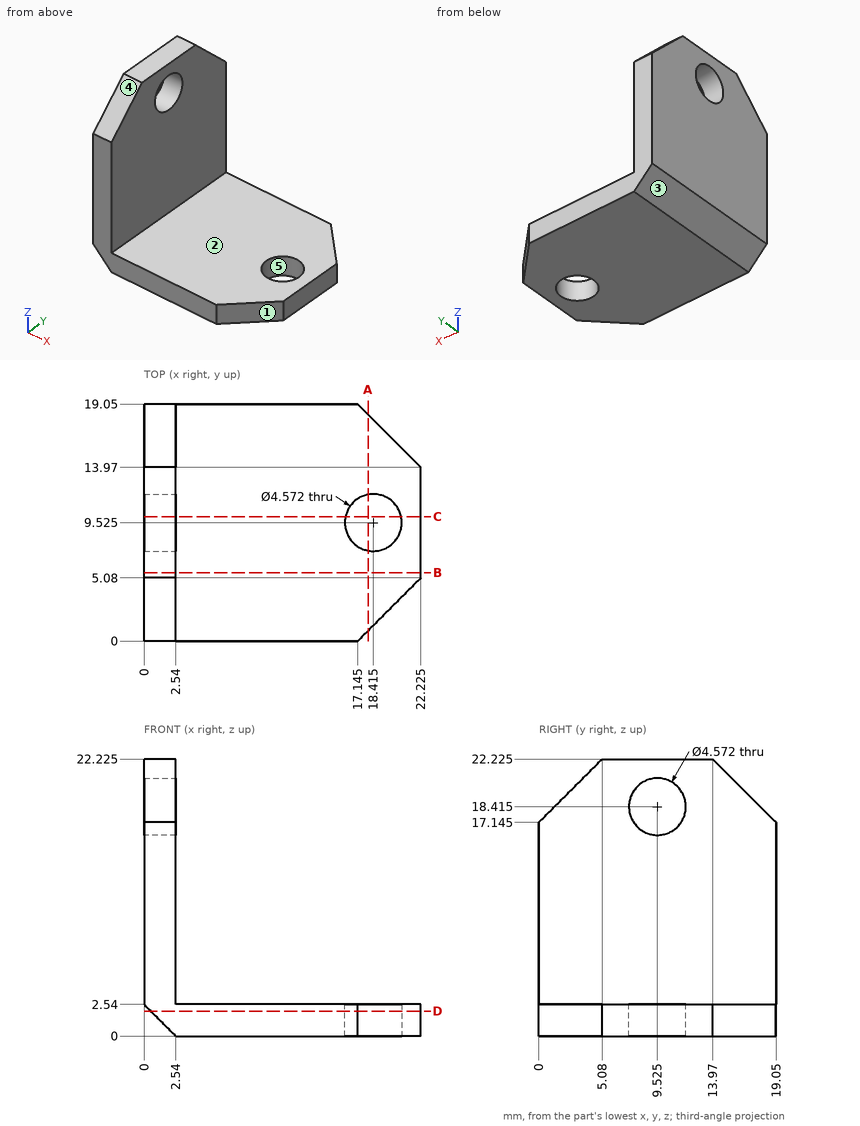
For this review, use the dimensioned drawing (mm, ordinates from the lowest corner) and the shaded views. A direction names the side the tool comes from. Give positions to 0.01 mm unless a question says otherwise; leave off trailing zeros. Order: outer loops, then holes, each group sorted by start corner. A loop starts at its lowest first (then second) coordinate and runs counter-clockwise, first axis right, second up. Notation, with made-up numbers: M -4,53 L 24,53 A21 ccw 24,77 Z; hole C -6,82 d11. An arc over 180 degrees is marked long. One line per question, with ' | ' between items. Start each with the question number.
1) Wall thickness on L1, parallel to Z at x = 8.75, y = 6; L2, parallel to X at y = 9.25, z = 1.5 (3 decimals): over which ranges is each line inside the solid? List them lowest first. Write a range as from..to.
2) Consider section C-C, the plane y = 10. Give the boundary of the cut face in (x, z) (3 decimals), then the cut area to 3 significant figures.
3) Clearance check with flat-ended pins moving along their axes: P1, Ø10, axis at x = 18.5, y = 15, coming from the +Z side; P2, Ø5.5, axis at y = 11.5, z = 8.5, coming from the +X side. State where each tip first meets the part, or that it passes through.
4) Consider section B-B, the plane y = 5.5. Give the boundary of the cut face in (x, z) (3 decimals).
5) Consider section D-D, the plane z = 2. Give the boundary of the cut face in (x, y) (3 decimals), then the cut area to 3 significant figures.
6) Consider section A-A, the plane x = 18. Give the boundary of the cut face in (y, z) (3 decimals).
7) Mouldability with a two-part tool opening along X and no side actions: class the marked faces 3, 4 and 5 as pulls with the +X half, pulls with the -X half, needs draft (parallel to the pull), parting line crosses it, or undercut.
8) For the marked faces 1 and 2, list the 3-axis set-ups (+Z, -Z, +X, -X, +Y, -Y) from which the entire face can be reached by the end or side of a thin tool; tool diameter is ignored.
Found:
1) L1: z = 0..2.54 | L2: x = 1.04..16.146, 20.684..22.225
2) outline: M 0,2.54 L 2.54,0 L 16.179,0 L 16.179,2.54 L 2.54,2.54 L 2.54,16.179 L 0,16.179 Z; M 0,20.651 L 2.54,20.651 L 2.54,22.225 L 0,22.225 Z; M 20.651,0 L 22.225,0 L 22.225,2.54 L 20.651,2.54 Z | area: 80.5 mm²
3) P1: stops at z = 2.54 | P2: stops at x = 2.54
4) outline: M 0,2.54 L 2.54,0 L 22.225,0 L 22.225,2.54 L 2.54,2.54 L 2.54,22.225 L 0,22.225 Z
5) outline: M 0.54,0 L 17.145,0 L 22.225,5.08 L 22.225,13.97 L 17.145,19.05 L 0.54,19.05 Z; hole C 18.415,9.525 d4.572 | area: 371 mm²
6) outline: M 0.855,0 L 7.277,0 L 7.277,2.54 L 0.855,2.54 Z; M 11.773,0 L 18.195,0 L 18.195,2.54 L 11.773,2.54 Z
7) face 3: pulls with the -X half | face 4: needs draft | face 5: undercut
8) face 1: +Z, -Z, +X, -Y | face 2: +Z, +X, +Y, -Y
